Check sheet for the drawn part. Datum: minimum x, y, z corner. Units: mm. A direction names the side the tool comes from. Round coordinates to 2 decimals unless told otherwise and drop trailing zeros. Write each loop counter-clockwise with the first axis right and the second up, starting at its lowest first coordinate (ties: lowest second). Pieces come first, ordered by that corner, then holes. Notation, with made-up numbers: M -16.5,17.5 L 40.5,17.5 A29 ccw 40.5,43.5 Z; hole C 60,17 d9. An arc over 180 degrees is marked long. One line per item, written item: value.
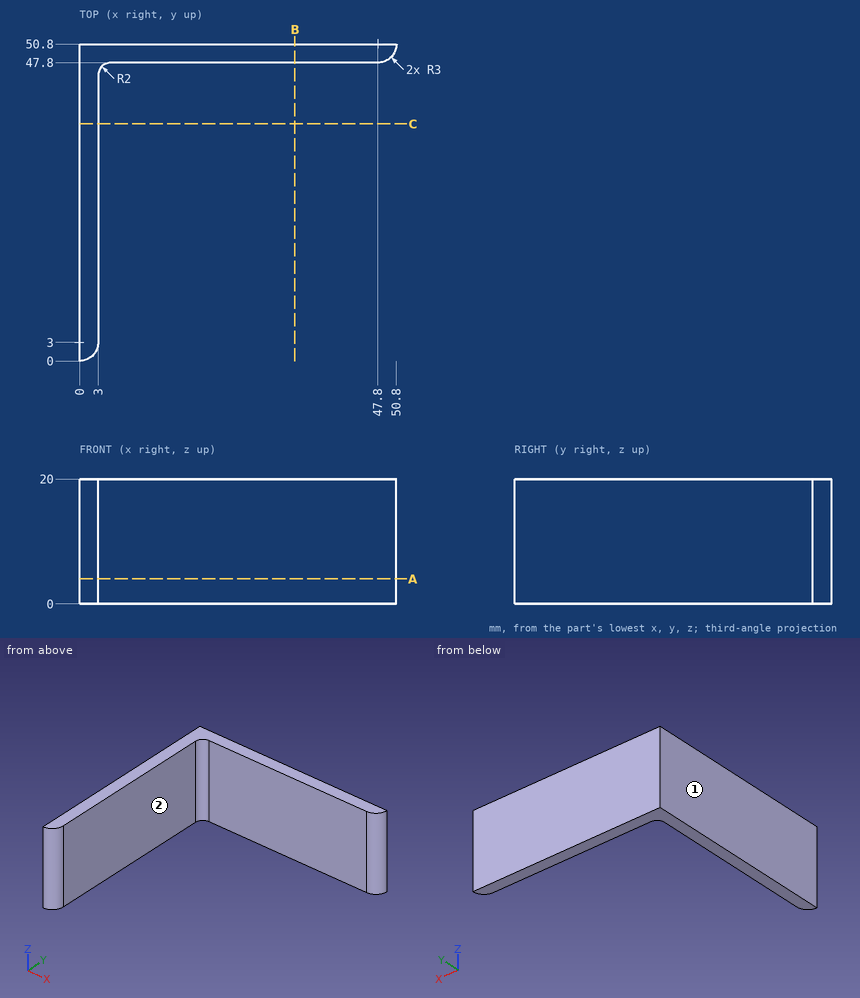
Q1. Sectioned sample at C-C on y = 38. Enter the section's corners in (x, z).
Completed:
outline: M 0,0 L 3,0 L 3,20 L 0,20 Z
Q2. Scan lines: line 1 (Y direction, x = 21.5, z = 7.75); line 2 (X direction, y = 6.5, z = 1); line 3 (Y direction, x = 48.5, z = 3.75). Record each from-to range of solid material in increasing order. Write a range as [from, to].
Completed:
line 1: [47.8, 50.8]
line 2: [0, 3]
line 3: [47.88, 50.8]
Q3. Sectioned sample at A-A on z = 4. Enter the section's corners in (x, y), and give its area (3 significant figures).
Completed:
outline: M 0,0 A3 ccw 3,3 L 3,45.8 A2 cw 5,47.8 L 47.8,47.8 A3 ccw 50.8,50.8 L 0,50.8 Z
area: 293 mm^2
Q4. Sectioned sample at B-B on x = 34.5. Enter the section's corners in (y, z).
Completed:
outline: M 47.8,0 L 50.8,0 L 50.8,20 L 47.8,20 Z
Q5. Depth check by flat-ended pin: P1, Ø3, axis at x = 6.5, z = 5, coming from the -Y side; P2, Ø4, axis at y = 6.5, z = 11, coming from the +X side. Enter the tip coordinate at first touch or a pass-through.
Completed:
P1: y = 47.8
P2: x = 3
Q6. Access from +Z, -Z, +X, -X, +Y, -Y to the whole of each face (thin tool, end or side, straight path). Record for the marked faces 1 and 2.
Completed:
face 1: +Z, -Z, -X, +Y, -Y
face 2: +Z, -Z, +X, -Y
